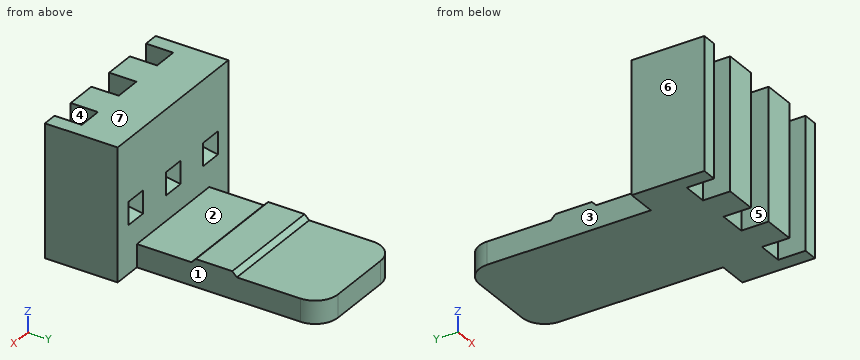
from build123d import *

# Parameters (mm, degrees)
EXTRUDE_1_DEPTH                  = 5.8
SKETCH_2_W                       = 4.9
SKETCH_2_H                       = 1
EXTRUDE_2_DEPTH                  = 8.2
SKETCH_3_W                       = 4.9
SKETCH_3_H                       = 2
EXTRUDE_3_DEPTH                  = 0.2
CHAMFER_1_SIZE                   = 0.2
FILLET_1_R                       = 1
SKETCH_4_W                       = 1
SKETCH_4_H                       = 1
CUT_EXTRUDE_1_DEPTH              = 0.5
CUT_EXTRUDE_1_DRAFT              = -44
PATTERN_LINEAR_1_COPY_1_SKETCH_W = 1
PATTERN_LINEAR_1_COPY_1_SKETCH_H = 1
PATTERN_LINEAR_1_COPY_1_DEPTH    = 0.5
PATTERN_LINEAR_1_COPY_1_DRAFT    = -44
PATTERN_LINEAR_1_COPY_2_SKETCH_W = 1
PATTERN_LINEAR_1_COPY_2_SKETCH_H = 1
PATTERN_LINEAR_1_COPY_2_DEPTH    = 0.5
PATTERN_LINEAR_1_COPY_2_DRAFT    = -44


with BuildPart() as part:
    # Эскиз1 → Бобышка-Вытянуть1 (new body)
    with BuildSketch(Plane.XY):
        Polygon((0, 0), (0, 3.2), (7.5, 3.2), (7.5, 0), (6.85, 0), (6.85, 1.2), (5.75, 1.2), (5.75, 0), (4.35, 0), (4.35, 1.2), (3.15, 1.2), (3.15, 0), (1.75, 0), (1.75, 1.2), (0.65, 1.2), (0.65, 0), align=None)
    extrude(amount=EXTRUDE_1_DEPTH)

    # Эскиз2 → Бобышка-Вытянуть2 (add)
    with BuildSketch(Plane(origin=(0, 3.2, 0), x_dir=(1, 0, 0), z_dir=(0, 1, 0))):
        with Locations((3.75, -0.5)):
            Rectangle(SKETCH_2_W, SKETCH_2_H)
    extrude(amount=EXTRUDE_2_DEPTH)

    # Эскиз3 → Бобышка-Вытянуть3 (add)
    with BuildSketch(Plane.XY.offset(1)):
        with Locations((3.75, 6.6)):
            Rectangle(SKETCH_3_W, SKETCH_3_H)
    extrude(amount=EXTRUDE_3_DEPTH)

    # Фаска1
    chamfer_1_edges = [part.edges().sort_by_distance(p)[0] for p in [
        (3.75, 5.6, 1.2),
        (3.75, 7.6, 1.2),
    ]]
    chamfer(chamfer_1_edges, length=CHAMFER_1_SIZE - 0.0001)  # a hair under: the kernel refuses the full size

    # Скругление1
    fillet_1_edges = [part.edges().sort_by_distance(p)[0] for p in [
        (1.3, 11.4, 0.5),
        (6.2, 11.4, 0.5),
    ]]
    fillet(fillet_1_edges, radius=FILLET_1_R)


with BuildPart() as cut_extrude_1_tool:
    # Эскиз4 → Вырез-Вытянуть1 (with draft: the straight prism first)
    with BuildSketch(Plane(origin=(0, 3.2, 0), x_dir=(1, 0, 0), z_dir=(0, 1, 0))):
        with Locations((1.2, -2.6)):
            Rectangle(SKETCH_4_W, SKETCH_4_H)
    extrude(amount=-CUT_EXTRUDE_1_DEPTH)
    # Вырез-Вытянуть1: the draft: its side faces are tilted about the plane it starts from
    cut_extrude_1_sides = [cut_extrude_1_tool.faces().sort_by_distance(p)[0] for p in [
        (0.7, 2.95, 2.6),
        (1.2, 2.95, 3.1),
        (1.7, 2.95, 2.6),
        (1.2, 2.95, 2.1),
    ]]
    draft(cut_extrude_1_sides, Plane(origin=(0, 3.2, 0), x_dir=(1, 0, 0), z_dir=(0, 1, 0)), CUT_EXTRUDE_1_DRAFT)


with BuildPart() as part_1:
    add(part.part)

    # Вырез-Вытянуть1: cut by cut_extrude_1_tool
    add(cut_extrude_1_tool.part, mode=Mode.SUBTRACT)


with BuildPart() as pattern_linear_1_copy_1_tool:
    # Линейный массив1 copy 1 sketch → Линейный массив1 copy 1 (with draft: the straight prism first)
    with BuildSketch(Plane(origin=(2.54, 3.2, 0), x_dir=(1, 0, 0), z_dir=(0, 1, 0))):
        with Locations((1.2, -2.6)):
            Rectangle(PATTERN_LINEAR_1_COPY_1_SKETCH_W, PATTERN_LINEAR_1_COPY_1_SKETCH_H)
    extrude(amount=-PATTERN_LINEAR_1_COPY_1_DEPTH)
    # Линейный массив1 copy 1: the draft: its side faces are tilted about the plane it starts from
    pattern_linear_1_copy_1_sides = [pattern_linear_1_copy_1_tool.faces().sort_by_distance(p)[0] for p in [
        (3.24, 2.95, 2.6),
        (3.74, 2.95, 3.1),
        (4.24, 2.95, 2.6),
        (3.74, 2.95, 2.1),
    ]]
    draft(pattern_linear_1_copy_1_sides, Plane(origin=(2.54, 3.2, 0), x_dir=(1, 0, 0), z_dir=(0, 1, 0)), PATTERN_LINEAR_1_COPY_1_DRAFT)


with BuildPart() as part_2:
    add(part_1.part)

    # Линейный массив1 copy 1: cut by pattern_linear_1_copy_1_tool
    add(pattern_linear_1_copy_1_tool.part, mode=Mode.SUBTRACT)


with BuildPart() as pattern_linear_1_copy_2_tool:
    # Линейный массив1 copy 2 sketch → Линейный массив1 copy 2 (with draft: the straight prism first)
    with BuildSketch(Plane(origin=(5.08, 3.2, 0), x_dir=(1, 0, 0), z_dir=(0, 1, 0))):
        with Locations((1.2, -2.6)):
            Rectangle(PATTERN_LINEAR_1_COPY_2_SKETCH_W, PATTERN_LINEAR_1_COPY_2_SKETCH_H)
    extrude(amount=-PATTERN_LINEAR_1_COPY_2_DEPTH)
    # Линейный массив1 copy 2: the draft: its side faces are tilted about the plane it starts from
    pattern_linear_1_copy_2_sides = [pattern_linear_1_copy_2_tool.faces().sort_by_distance(p)[0] for p in [
        (5.78, 2.95, 2.6),
        (6.28, 2.95, 3.1),
        (6.78, 2.95, 2.6),
        (6.28, 2.95, 2.1),
    ]]
    draft(pattern_linear_1_copy_2_sides, Plane(origin=(5.08, 3.2, 0), x_dir=(1, 0, 0), z_dir=(0, 1, 0)), PATTERN_LINEAR_1_COPY_2_DRAFT)


with BuildPart() as part_3:
    add(part_2.part)

    # Линейный массив1 copy 2: cut by pattern_linear_1_copy_2_tool
    add(pattern_linear_1_copy_2_tool.part, mode=Mode.SUBTRACT)


solid = part_3.part
Design review of the part built by this model. Coordinates are the model's own, in mm. Face numbers are marked on the shaded views. A direction names the side the tool comes from. Coordinates: 2 decimals unless noted, no trailing zeros. Loops run counter-clockwise (first coordinate to the right, second up) from the corner with the lowest first, then second, coordinate; pieces in that order, holes last. Notation, with made-up numbers: M -10.75,26.25 L 23.25,26.25 A12 ccw 23.25,38.25 Z; hole C -15.5,-37.5 d4. An arc over 180 degrees is marked long. Answer as CSV lines item,"result".
Item 1: Add section C-C on y = 10.25. State the section outline as (x, z) points.
Answer list:
outline,"M 1.3,0 L 6.2,0 L 6.2,1 L 1.3,1 Z"
Item 2: Add section A-A on z = 3.4. State the section outline as (x, y) points.
Answer list:
outline,"M 0,0 L 0.65,0 L 0.65,1.2 L 1.75,1.2 L 1.75,0 L 3.15,0 L 3.15,1.2 L 4.35,1.2 L 4.35,0 L 5.75,0 L 5.75,1.2 L 6.85,1.2 L 6.85,0 L 7.5,0 L 7.5,3.2 L 0,3.2 Z"
Item 3: Machinability: for the marked faces 1, 2, 3 and 4, which of the approach directions +Z, -Z, +X, -X, +Y, -Y give a long, thin tool a straight path to every point of the face, cutting with its end or side? Answer none if there is none.
Answer list:
face 1,"+Z, -Z, +X, +Y"
face 2,"+Z, +X, -X"
face 3,"+Z, -Z, -X, +Y"
face 4,"+Z, -Z, -Y"
Item 4: The part is to be moulded in two halves that separate along X. For the marked faces 5, 6 and 7, say which applies: pulls with the +X half, pulls with the -X half, needs draft (parallel to the pull), parting line crosses it, or undercut.
Answer list:
face 5,"undercut"
face 6,"pulls with the -X half"
face 7,"needs draft"
Item 5: For P1, Ø0.7, axis at x = 2.5, y = 4.5, coming from the +Z side; P2, Ø0.6, axis at y = 0.5, z = 2.5, coming from the -X side; P3, Ø4, axis at x = 3.5, y = 9.5, coming from the +Z side; P4, Ø1.8, axis at x = 4.5, y = 6.5, coming from the +Z side, all flat-tipped, find the tip position at first contact; note any pin that passes through.
Answer list:
P1,"z = 1"
P2,"x = 0"
P3,"z = 1.1"
P4,"z = 1.2"
Item 6: For probe 1 along X at (y, z) = (1, 4.8); probe 2 along Z at (x, y) = (6, 4); probe 3 along X at (y, z) = (9.25, 0.7), list the stretches that pass through material, from the lowest coordinate up.
Answer list:
probe 1,"0 to 0.65, 1.75 to 3.15, 4.35 to 5.75, 6.85 to 7.5"
probe 2,"0 to 1"
probe 3,"1.3 to 6.2"
Item 7: Add section D-D on z = 0.5. State the section outline as (x, y) points.
Answer list:
outline,"M 0,0 L 0.65,0 L 0.65,1.2 L 1.75,1.2 L 1.75,0 L 3.15,0 L 3.15,1.2 L 4.35,1.2 L 4.35,0 L 5.75,0 L 5.75,1.2 L 6.85,1.2 L 6.85,0 L 7.5,0 L 7.5,3.2 L 6.2,3.2 L 6.2,10.4 A1 ccw 5.2,11.4 L 2.3,11.4 A1 ccw 1.3,10.4 L 1.3,3.2 L 0,3.2 Z"
